Autodesk Inventor part; units mm, degrees
ref_plane "YZ Plane" through (0, 0, 0) normal (1, 0, 0) x (0, 1, 0)
ref_plane "XZ Plane" through (0, 0, 0) normal (0, 1, 0) x (-1, 0, 0)
sketch "Sketch1" plane through (0, 0, 0) normal (0, 0, 1) x (1, 0, 0)
  circle A0 centre (0, 0) radius 2.25
  line L0 (-4, 3) -> (3, 3)
  line L1 (3, 3) -> (3, -4)
  line L2 (3, -4) -> (-4, -4)
  line L3 (-4, -4) -> (-4, 3)
  line L4 (-4, 3) -> (-5.5, 3)
  line L5 (-5.5, 3) -> (-5.5, -5.5)
  line L6 (-5.5, -5.5) -> (-4, -5.5)
  line L7 (-4, -5.5) -> (-4, 3)
  line L8 (3, -4) -> (-4, -4)
  line L9 (-4, -4) -> (-4, -5.5)
  line L10 (-4, -5.5) -> (3, -5.5)
  line L11 (3, -5.5) -> (3, -4)
  dimension "d0" = 4.5
  dimension "d1" = 4
  dimension "d2" = 4
  dimension "d3" = 3
  dimension "d5" = 3
  dimension "d6" = 1.5
  dimension "d7" = 1.5
extrude "Extrusion1" add sketch "Sketch1" along normal blind 1.5
extrude "Extrusion2" add sketch "Sketch1" along normal blind 29.5 contours L3 L7 L6 L5 L4 | L2 L11 L10 L7
ref_plane "Work Plane2" through (0, 0, 15.5) normal (0, 0, 1) x (1, 0, 0)
mirror "Mirror2" about plane through (0, 0, 15.5) normal (0, 0, 1) of "Extrusion1"
sketch "Sketch2" plane through (-4, -4, 1.5) normal (0, 1, 0) x (1, 0, 0)
  line L0 (7, 0) -> (7, -28)
  line L1 (0, 0) -> (7, 0)
  line L2 (7, 0) -> (7, -3.5)
  line L3 (7, -3.5) -> (0, -3.5)
  line L4 (0, -3.5) -> (0, 0)
  point P0 (4, 1.5)
  dimension "d13" = 3.5
extrude "Extrusion3" cut sketch "Sketch2" against normal blind 10
mirror "Mirror3" about plane through (0, 0, 15.5) normal (0, 0, 1) of "Extrusion3"
properties part number "Lifter"
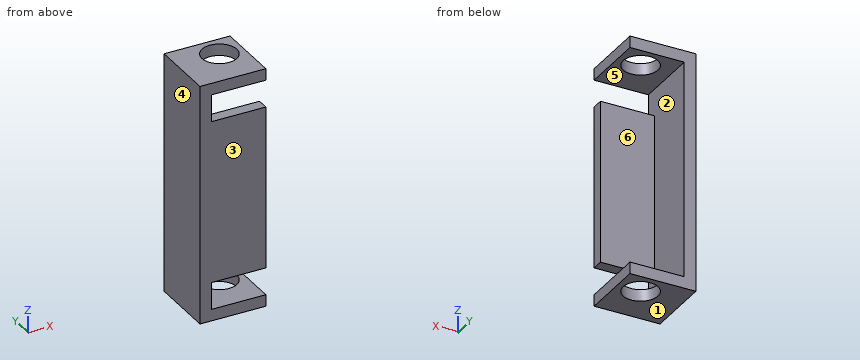
Could you check a few things on this model? Use its own coordinates, in mm. Face numbers are marked on the shaded views. A direction names the side the tool comes from. Coordinates: 2 decimals unless noted, no trailing zeros. Loops run counter-clockwise (first coordinate to the right, second up) from the corner with the lowest first, then second, coordinate; pieces in that order, holes last.
1. Imagine slicing it at A-A (y = 0). Please give me the cut outline in (x, z), and give its area (3 significant figures).
2. Imagine slicing it at B-B (x = -3). Please give me the cut outline in (y, z), and give its area (3 significant figures).
3. I need wall thicknesses on L1, parallel to Y at x = 0, z = 29.95; L2, parallel to Z at x = 1, y = -3.5; L3, parallel to Z at x = 1.5, y = -4.5. Which ranges of each line are inside material? Lowest first, please.
4. For the marked faces 4, 5 and 6, which set-ups out of +Z, -Z, +X, -X, +Y, -Y let a thin tool reach every point of the face, with its end or its side?
5. For P1, Ø1.6, axis at x = -0.5, y = -5, coming from the -Z side; P2, Ø3.5, axis at x = -1, z = 17, coming from the +Y side; P3, Ø3, axis at y = 0.5, z = 15.5, coming from the +X side, each with a flat end and sliding along its axis, tell me the tip position at first contact or that it passes through.
6. We'd pull the mould along Z, two halves only. Please class the marked faces 1, 2 and 3: released by +Z, released by -Z, zero draft, split by the parting line, or undercut.
7. Imagine slicing it at C-C (x = 0). Please give me the cut outline in (y, z).
8. Imagine slicing it at D-D (z = 14.5). Please give me the cut outline in (x, y).
Computed values:
1. outline: (-5.5, 0) - (-2.25, 0) - (-2.25, 1.5) - (-4, 1.5) - (-4, 29.5) - (-2.25, 29.5) - (-2.25, 31) - (-5.5, 31) - close; (2.25, 0) - (3, 0) - (3, 1.5) - (2.25, 1.5) - close; (2.25, 29.5) - (3, 29.5) - (3, 31) - (2.25, 31) - close
1. area: 54.0 mm2
2. outline: (-5.5, 0) - (3, 0) - (3, 1.5) - (-5.5, 1.5) - close; (-5.5, 5) - (-4, 5) - (-4, 26) - (-5.5, 26) - close; (-5.5, 29.5) - (3, 29.5) - (3, 31) - (-5.5, 31) - close
2. area: 57.0 mm2
3. L1: y = -5.5 to -2.25, 2.25 to 3
3. L2: z = 0 to 1.5, 29.5 to 31
3. L3: z = 0 to 1.5, 5 to 26, 29.5 to 31
4. face 4: +Z, -Z, -X, +Y, -Y
4. face 5: +X, +Y, -Y
4. face 6: +X, +Y
5. P1: stops at z = 0
5. P2: stops at y = -4
5. P3: stops at x = -4
6. face 1: released by -Z
6. face 2: undercut
6. face 3: zero draft
7. outline: (-5.5, 0) - (-2.25, 0) - (-2.25, 1.5) - (-5.5, 1.5) - close; (-5.5, 5) - (-4, 5) - (-4, 26) - (-5.5, 26) - close; (-5.5, 29.5) - (-2.25, 29.5) - (-2.25, 31) - (-5.5, 31) - close; (2.25, 0) - (3, 0) - (3, 1.5) - (2.25, 1.5) - close; (2.25, 29.5) - (3, 29.5) - (3, 31) - (2.25, 31) - close
8. outline: (-5.5, -5.5) - (3, -5.5) - (3, -4) - (-4, -4) - (-4, 3) - (-5.5, 3) - close
